For this review, take the finished solid that the model builds, in its own axes (mm). A direction names the side the tool comes from. Give positions to 0.01 mm unless a question says otherwise; leave off trailing zeros. Loops run counter-clockwise (first coordinate to the right, second up) from the corner with the lowest first, then second, coordinate; pieces in that order, holes last. Notation, with made-up numbers: (13.5, -11.5) -> (20.5, -11.5) arc R22 ccw to (20.5, 3.5) -> close; hole circle Ø10 at (-7, 21.5). An arc over 180 degrees is marked (long way). Answer as CSV lines item,"result". Start each with the question number.
Item 1: Clearance check with flat-ended pins moving along their axes: P1, Ø5, axis at y = -6, z = 8.5, coming from the -X side; P2, Ø7, axis at x = 0, y = 0, coming from the +Z side; P3, Ø1.5, axis at x = -5.5, y = -4.5, coming from the -Z side; P4, Ø2, axis at x = -3, z = 4.5, coming from the +Y side. State where each tip first meets the part, or that it passes through.
Item 2: Add section A-A on y = 0. State the section outline as (x, z) points, plus the area to 3 significant figures.
Item 3: The part is to be moulded in two halves that separate along X. For faces 4 (the face through (-7, 3, -3)), 5 (the face through (-3.304, 6.352, 18.465)), 6 (the face through (-1.07, 8.13, 8.89)), say which applies: +X half, -X half, draft (parallel to the pull), parting line (faces both ways), or undercut.
Item 4: Add section D-D on z = 16.5. State the section outline as (x, y) points.
Item 5: Add section C-C on z = -0.5. State the section outline as (x, y) points, plus the area to 3 significant figures.
Item 6: For L1, parallel to Y at x = 0, z = 19.8; L2, parallel to Y at x = 0, z = 12, list the stretches that pass through material, from the lowest coordinate up. Write a range as from..to.
Item 7: Machinability: for faces 1 (the face through (0, 3, 15)), 2 (the face through (1.55, -6.99, -0.54)), 3 (the face through (-6.633, -6.083, -1.521)), which of the approach directions +Z, -Z, +X, -X, +Y, -Y give a long, thin tool a straight path to every point of the face, cutting with its end or side? Answer none if there is none.
```python
from build123d import *

# Parameters (mm, degrees)
SZKIC1_R                    = 8.2
SZKIC1_R_2                  = 2.2
DODANIE_WYCI_GNI_CIE6_DEPTH = 18
SZKIC6_R                    = 9
SZKIC6_R_2                  = 2.2
DODANIE_WYCI_GNI_CIE7_DEPTH = 3
DODANIE_WYCI_GNI_CIE8_START = 3
SZKIC7_R                    = 9
SZKIC7_R_2                  = 2.2
DODANIE_WYCI_GNI_CIE8_DEPTH = 3
SZKIC8_R                    = 7.16
WYTNIJ_WYCI_GNI_CIE2_DEPTH  = 6
WYTNIJ_WYCI_GNI_CIE3_START  = -6
SZKIC9_R                    = 7.16
SZKIC9_R_2                  = 2.2
WYTNIJ_WYCI_GNI_CIE3_DEPTH  = 6
ZAOKR_GLENIE2_R             = 1
ZAOKR_GLENIE3_R             = 1
ZAOKR_GLENIE4_R             = 1


with BuildPart() as part:
    # Szkic1 → Dodanie-wyciągnięcie6 (new body)
    with BuildSketch(Plane.XY):
        Circle(SZKIC1_R)
        Circle(SZKIC1_R_2, mode=Mode.SUBTRACT)
    extrude(amount=DODANIE_WYCI_GNI_CIE6_DEPTH)

    # Szkic6 → Dodanie-wyciągnięcie7 (add)
    with BuildSketch(Plane.XY.offset(18)):
        Circle(SZKIC6_R)
        Circle(SZKIC6_R_2, mode=Mode.SUBTRACT)
    extrude(amount=DODANIE_WYCI_GNI_CIE7_DEPTH)

    # Szkic7 → Dodanie-wyciągnięcie8 (add)
    with BuildSketch(Plane(origin=(0, 0, 0), x_dir=(-1, 0, 0), z_dir=(0, 0, -1)).offset(DODANIE_WYCI_GNI_CIE8_START)):
        with Locations(Location((0, 0, 0), (0, 0, 180))):
            Circle(SZKIC7_R)
        Circle(SZKIC7_R_2, mode=Mode.SUBTRACT)
    extrude(amount=-DODANIE_WYCI_GNI_CIE8_DEPTH)

    # Szkic8 → Wytnij-wyciągnięcie2 (cut)
    with BuildSketch(Plane(origin=(0, 0, -3), x_dir=(-1, 0, 0), z_dir=(0, 0, -1))):
        Circle(SZKIC8_R)
    extrude(amount=-WYTNIJ_WYCI_GNI_CIE2_DEPTH, mode=Mode.SUBTRACT)

    # Szkic9 → Wytnij-wyciągnięcie3 (cut)
    with BuildSketch(Plane.XY.offset(21).offset(WYTNIJ_WYCI_GNI_CIE3_START)):
        with Locations(Location((0, 0, 0), (0, 0, 180))):
            Circle(SZKIC9_R)
        with Locations(Location((0, 0, 0), (0, 0, 180))):
            Circle(SZKIC9_R_2, mode=Mode.SUBTRACT)
    extrude(amount=WYTNIJ_WYCI_GNI_CIE3_DEPTH, mode=Mode.SUBTRACT)

    # Zaokrąglenie2
    # the kernel refuses this fillet: 1 mm, written as the material it adds along each edge
    with BuildSketch(Plane(origin=(0, 0, 0), x_dir=(1, 0, 0), z_dir=(0, -1, 0))) as zaokr_glenie2_piece_1:
        with BuildLine():
            CenterArc((9.2, 0.979795897), ZAOKR_GLENIE2_R, 180, 78.463040967)
            Line((9, 0), (8.996, -0.019595918))
            ThreePointArc((8.996, -0.019595918), (8.6, -0.02), (8.2, -0.02))
            Line((8.2, -0.02), (8.18, 0))
            Line((8.18, 0), (8.18, 0.979795897))
            Line((8.18, 0.979795897), (8.2, 0.979795897))
        make_face()
    revolve(axis=Axis((0, 0, 0), (0, 0, 1)))
    with BuildSketch(Plane(origin=(0, 0, 18), x_dir=(1, 0, 0), z_dir=(0, -1, 0))) as zaokr_glenie2_piece_2:
        with BuildLine():
            CenterArc((9.2, -0.979795897), ZAOKR_GLENIE2_R, 101.536959033, 78.463040967)
            Line((9, 0), (8.996, 0.019595918))
            ThreePointArc((8.996, 0.019595918), (8.6, 0.02), (8.2, 0.02))
            Line((8.2, 0.02), (8.18, 0))
            Line((8.18, 0), (8.18, -0.979795897))
            Line((8.18, -0.979795897), (8.2, -0.979795897))
        make_face()
    revolve(axis=Axis((0, 0, 18), (0, 0, 1)))

    # Zaokrąglenie3
    zaokr_glenie3_edges = [part.edges().sort_by_distance(p)[0] for p in [
        (7.16, 0, 3),
    ]]
    fillet(zaokr_glenie3_edges, radius=ZAOKR_GLENIE3_R)

    # Zaokrąglenie4
    zaokr_glenie4_edges = [part.edges().sort_by_distance(p)[0] for p in [
        (7.16, 0, 15),
    ]]
    fillet(zaokr_glenie4_edges, radius=ZAOKR_GLENIE4_R)


solid = part.part
```
Computed values:
1,P1,"x = -7.42"
1,P2,"z = 15"
1,P3,"z = -3"
1,P4,"y = 7.95"
2,outline,"(-9, -3) -> (-7.16, -3) -> (-7.16, 2) arc R1 cw to (-6.16, 3) -> (-2.2, 3) -> (-2.2, 15) -> (-6.16, 15) arc R1 cw to (-7.16, 16) -> (-7.16, 21) -> (-9, 21) -> (-9, 18) arc R1 cw to (-8.2, 17.02) -> (-8.2, 0.98) arc R1 cw to (-9, 0) -> close; (2.2, 3) -> (6.16, 3) arc R1 cw to (7.16, 2) -> (7.16, -3) -> (9, -3) -> (9, 0) arc R1 cw to (8.2, 0.98) -> (8.2, 17.02) arc R1 cw to (9, 18) -> (9, 21) -> (7.16, 21) -> (7.16, 16) arc R1 cw to (6.16, 15) -> (2.2, 15) -> close"
2,area,"180 mm²"
3,face 4,"draft"
3,face 5,"undercut"
3,face 6,"parting line"
4,outline,"circle Ø16.4 at (0, 0); hole circle Ø14.32 at (0, 0)"
5,outline,"circle Ø18 at (0, 0); hole circle Ø14.32 at (0, 0)"
5,area,"93.4 mm²"
6,L1,"-9..-7.16, 7.16..9"
6,L2,"-8.2..-2.2, 2.2..8.2"
7,face 1,"+Z"
7,face 2,"-Z"
7,face 3,"+Z, -Z"
